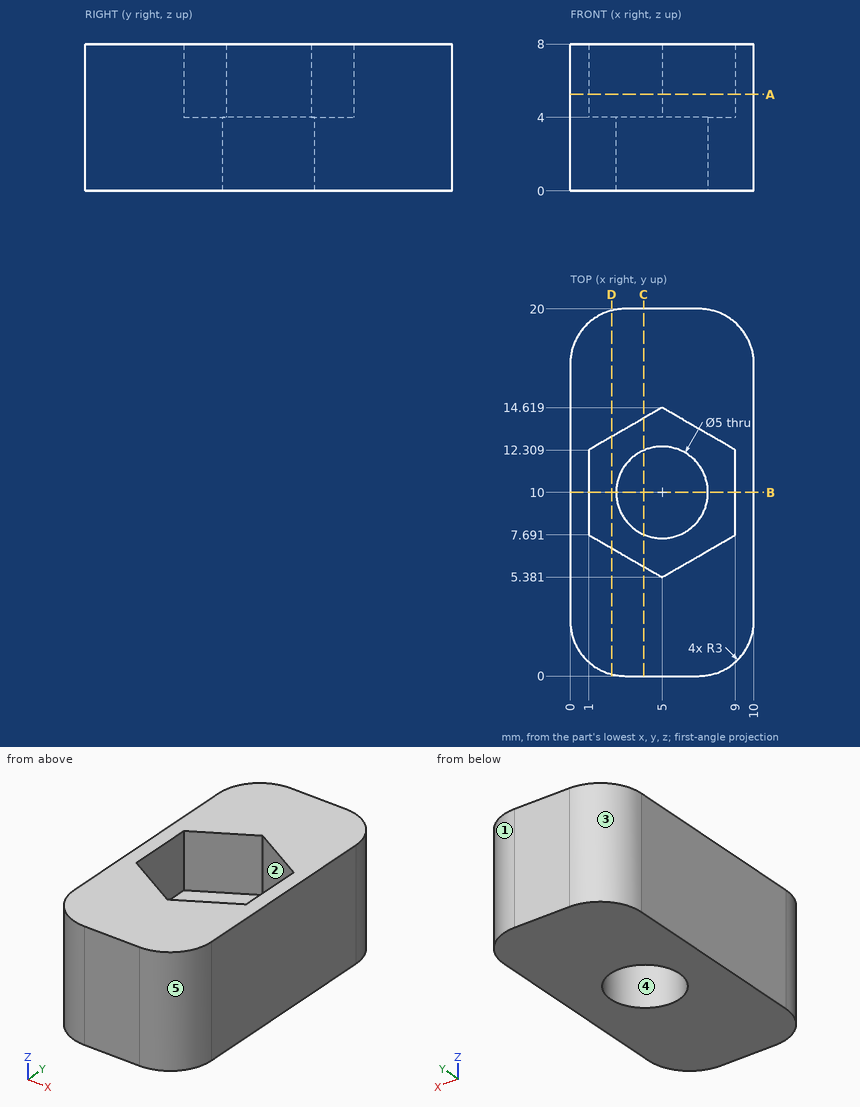
Verification items for this drawing (mm, ordinates from the low corner). A direction names the side the tool comes from. Give positions to 0.01 mm unless a question says otherwise; leave off trailing zeros. Loops run counter-clockwise (first coordinate to the right, second up) from the corner with the lowest first, then second, coordinate; pieces in that order, holes last. Notation, with made-up numbers: M 63.5,22 L 74.5,22 A25 cw 74.5,56 Z; hole C -2.75,-3 d11. An arc over 180 degrees is marked long. Answer as a JSON object with one key per item and string values. Group by question number.
Item 1: Sectioned sample at D-D on x = 2.25. Record the boundary of the cut face in (y, z) (1 decimal), plus the area to 3 significant figures.
Item 2: Access from +Z, -Z, +X, -X, +Y, -Y to the whole of each face (thin tool, end or side, straight path). Record for the marked faces 1 and 2.
Item 3: Gauge pin test, flat ends, axial feed: pin 1 (1.2 mm diameter, centred on y = 10.5, z = 5.5, fed in from -X); pin 2 (2.5 mm diameter, centred on x = 4, y = 8, fed in from +Z); pin 3 (1.5 mm diameter, centred on x = 2, z = 3, fed in from +Y). Record the tip position at first contact, or that the pin passes through.
Item 4: Material ranges on L1, parallel to X at y = 12.25, z = 7; L2, parallel to Y at x = 5, z = 2.95; L3, parallel to Z at x = 7.5, y = 7.25, recorded low to high.
Item 5: Sectioned sample at B-B on y = 10. Record the boundary of the cut face in (x, z).
Item 6: Sectioned sample at C-C on x = 4. Record the boundary of the cut face in (y, z), plus the area to 3 significant figures.
Item 7: Mould release check, pull along Y, two halves, no side actions. Record for the marked faces 3, 4 and 5: pulls with the +Y half, pulls with the -Y half, needs draft (parallel to the pull), parting line crosses it, or undercut.
Item 8: Sectioned sample at A-A on z = 5.25. Record the boundary of the cut face in (x, y), plus the area to 3 significant figures.
Findings below:
{
 "1": {"outline": "M 0.1,0 L 19.9,0 L 19.9,8 L 13,8 L 13,4 L 7,4 L 7,8 L 0.1,8 Z", "area": "134 mm2"},
 "2": {"face 1": "+Z, -Z, +X, +Y", "face 2": "+Z"},
 "3": {"pin 1": "x = 0", "pin 2": "z = 4", "pin 3": "y = 19.99"},
 "4": {"L1": "0 to 1, 9 to 10", "L2": "0 to 7.5, 12.5 to 20", "L3": "0 to 4"},
 "5": {"outline": "M 0,0 L 2.5,0 L 2.5,4 L 1,4 L 1,8 L 0,8 Z; M 7.5,0 L 10,0 L 10,8 L 9,8 L 9,4 L 7.5,4 Z"},
 "6": {"outline": "M 0,0 L 7.71,0 L 7.71,4 L 5.96,4 L 5.96,8 L 0,8 Z; M 12.29,0 L 20,0 L 20,8 L 14.04,8 L 14.04,4 L 12.29,4 Z", "area": "109 mm2"},
 "7": {"face 3": "pulls with the +Y half", "face 4": "undercut", "face 5": "pulls with the -Y half"},
 "8": {"outline": "M 0,3 A3 ccw 3,0 L 7,0 A3 ccw 10,3 L 10,17 A3 ccw 7,20 L 3,20 A3 ccw 0,17 Z; hole M 1,7.69 L 5,5.38 L 9,7.69 L 9,12.31 L 5,14.62 L 1,12.31 Z", "area": "137 mm2"}
}
